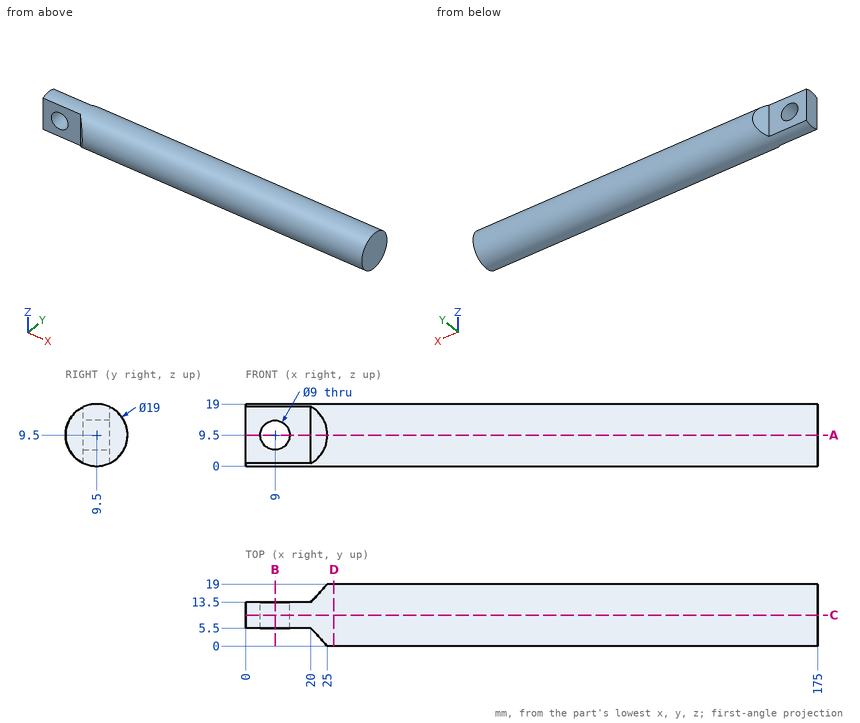
For this review, use the dimensioned drawing (mm, ordinates from the lowest corner) and the shaded views. Coordinates: 2 decimals unless noted, no trailing zeros. Order: outer loops, then holes, each group sorted by start corner. A loop starts at its lowest first (then second) coordinate and runs counter-clockwise, first axis right, second up. Notation, with made-up numbers: (70.25, 39) - (97.25, 39) arc R36 ccw to (97.25, 77) - close; hole circle Ø5 at (32.25, 20.25). An arc over 180 degrees is marked (long way). Use one line per item in the form item = value.
Q1. Consider section B-B (x = 9). Give the boundary of the cut face in (y, z).
Checked values:
outline = (5.5, 0.88) arc R9.5 ccw to (13.5, 0.88) - (13.5, 5) - (5.5, 5) - close; (5.5, 14) - (13.5, 14) - (13.5, 18.12) arc R9.5 ccw to (5.5, 18.12) - close
Q2. For P1, Ø2, axis at x = 83, z = 16.5, coming from the +Y side; P2, Ø3, axis at x = 104, z = 2.5, coming from the +Y side; P3, Ø5.5, axis at x = 9, z = 9.5, coming from the -Y side; P4, Ø3, axis at x = 59, y = 4.5, coming from the -Z side, all flat-tipped, find the tip position at first contact; note any pin that passes through.
Checked values:
P1 = 16.87
P2 = 17.25
P3 = through
P4 = 0.67
Q3. Consider section D-D (x = 27). Give the boundary of the cut face in (y, z).
Checked values:
outline = circle Ø19 at (9.5, 9.5)
Q4. Consider section A-A (z = 9.5). Give the boundary of the cut face in (x, y).
Checked values:
outline = (0, 5.5) - (4.5, 5.5) - (4.5, 13.5) - (0, 13.5) - close; (13.5, 5.5) - (20, 5.5) - (25, 0) - (175, 0) - (175, 19) - (25, 19) - (20, 13.5) - (13.5, 13.5) - close
Q5. Consider section C-C (y = 9.5). Give the boundary of the cut face in (x, z), then the cut area to 3 significant figures.
Checked values:
outline = (0, 0) - (175, 0) - (175, 19) - (0, 19) - close; hole circle Ø9 at (9, 9.5)
area = 3,260 mm2
Q6. For probe 1 along X at (y, z) = (10.5, 9.5); probe 2 along Y at (x, z) = (146.5, 5.5), list the stretches that pass through material, from the lowest coordinate up. Write a range as from..to.
Checked values:
probe_1 = 0..4.5, 13.5..175
probe_2 = 0.88..18.12
